Check sheet for the modelled part. Datum: model origin and axes. Units: mm. Face numbers are marked on the shaded views. A direction names the side the tool comes from. Give positions to 0.01 mm unless a question says otherwise; leave off trailing zeros. Order: outer loops, then holes, each group sorted by start corner. A loop starts at its lowest first (then second) coordinate and runs counter-clockwise, first axis right, second up.
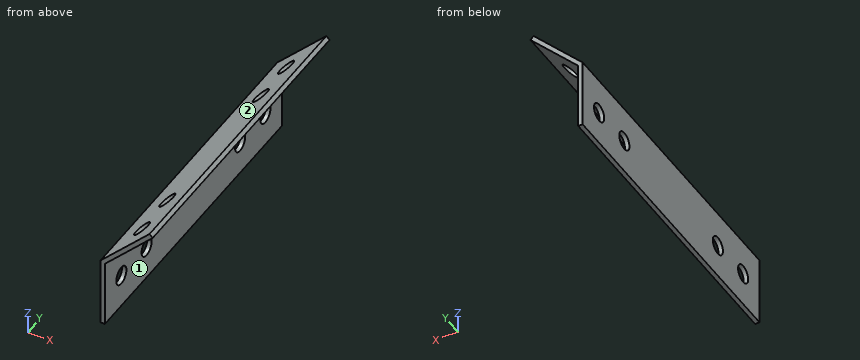
from build123d import *

# Parameters (mm, degrees)
EXTRUSION1_DEPTH = 70
EXTRUSION2_REACH = 3
ESQUISSE2_R      = 2
EXTRUSION3_REACH = 10.707
ESQUISSE3_R      = 2


with BuildPart() as part:
    # Esquisse1 → Extrusion1 (new body)
    with BuildSketch(Plane(origin=(0, 0, 0), x_dir=(1, 0, 0), z_dir=(0, 1, 0))):
        Polygon((0, 0), (0, 15.414213562), (1, 15.414213562), (1, 0.414213562), (11.606601718, -10.192388155), (10.899494937, -10.899494937), align=None)
    extrude(amount=EXTRUSION1_DEPTH)

    # Esquisse2 → Extrusion2 (cut, up to next)
    with BuildSketch(Plane(origin=(1, 0, 0), x_dir=(0, 0, -1), z_dir=(1, 0, 0)), mode=Mode.PRIVATE) as extrusion2_sk1:
        with Locations((7.914213562, 16.5)):
            Circle(ESQUISSE2_R)
    extrusion2_tool1 = extrude(extrusion2_sk1.sketch, amount=-EXTRUSION2_REACH, mode=Mode.PRIVATE) & part.part
    add(extrusion2_tool1.solids().sort_by_distance((1, 16.5, -7.914214))[0], mode=Mode.SUBTRACT)
    # Esquisse2 → Extrusion2 (cut, up to next)
    with BuildSketch(Plane(origin=(1, 0, 0), x_dir=(0, 0, -1), z_dir=(1, 0, 0)), mode=Mode.PRIVATE) as extrusion2_sk2:
        with Locations((7.914213562, 6.5)):
            Circle(ESQUISSE2_R)
    extrusion2_tool2 = extrude(extrusion2_sk2.sketch, amount=-EXTRUSION2_REACH, mode=Mode.PRIVATE) & part.part
    add(extrusion2_tool2.solids().sort_by_distance((1, 6.5, -7.914214))[0], mode=Mode.SUBTRACT)
    # Esquisse2 → Extrusion2 (cut, up to next)
    with BuildSketch(Plane(origin=(1, 0, 0), x_dir=(0, 0, -1), z_dir=(1, 0, 0)), mode=Mode.PRIVATE) as extrusion2_sk3:
        with Locations((7.914213562, 53.5)):
            Circle(ESQUISSE2_R)
    extrusion2_tool3 = extrude(extrusion2_sk3.sketch, amount=-EXTRUSION2_REACH, mode=Mode.PRIVATE) & part.part
    add(extrusion2_tool3.solids().sort_by_distance((1, 53.5, -7.914214))[0], mode=Mode.SUBTRACT)
    # Esquisse2 → Extrusion2 (cut, up to next)
    with BuildSketch(Plane(origin=(1, 0, 0), x_dir=(0, 0, -1), z_dir=(1, 0, 0)), mode=Mode.PRIVATE) as extrusion2_sk4:
        with Locations((7.914213562, 63.5)):
            Circle(ESQUISSE2_R)
    extrusion2_tool4 = extrude(extrusion2_sk4.sketch, amount=-EXTRUSION2_REACH, mode=Mode.PRIVATE) & part.part
    add(extrusion2_tool4.solids().sort_by_distance((1, 63.5, -7.914214))[0], mode=Mode.SUBTRACT)

    # Esquisse3 → Extrusion3 (cut, up to next)
    with BuildSketch(Plane(origin=(0.707106781, 0, -0.707106781), x_dir=(-0.707106781, 0, -0.707106781), z_dir=(0.707106781, 0, -0.707106781)), mode=Mode.PRIVATE) as extrusion3_sk1:
        with Locations((-7.914213562, 53.5)):
            Circle(ESQUISSE3_R)
    extrusion3_tool1 = extrude(extrusion3_sk1.sketch, amount=-EXTRUSION3_REACH, mode=Mode.PRIVATE) & part.part
    add(extrusion3_tool1.solids().sort_by_distance((6.303301, 53.5, 4.889087))[0], mode=Mode.SUBTRACT)
    # Esquisse3 → Extrusion3 (cut, up to next)
    with BuildSketch(Plane(origin=(0.707106781, 0, -0.707106781), x_dir=(-0.707106781, 0, -0.707106781), z_dir=(0.707106781, 0, -0.707106781)), mode=Mode.PRIVATE) as extrusion3_sk2:
        with Locations((-7.914213562, 63.5)):
            Circle(ESQUISSE3_R)
    extrusion3_tool2 = extrude(extrusion3_sk2.sketch, amount=-EXTRUSION3_REACH, mode=Mode.PRIVATE) & part.part
    add(extrusion3_tool2.solids().sort_by_distance((6.303301, 63.5, 4.889087))[0], mode=Mode.SUBTRACT)
    # Esquisse3 → Extrusion3 (cut, up to next)
    with BuildSketch(Plane(origin=(0.707106781, 0, -0.707106781), x_dir=(-0.707106781, 0, -0.707106781), z_dir=(0.707106781, 0, -0.707106781)), mode=Mode.PRIVATE) as extrusion3_sk3:
        with Locations((-7.914213562, 6.5)):
            Circle(ESQUISSE3_R)
    extrusion3_tool3 = extrude(extrusion3_sk3.sketch, amount=-EXTRUSION3_REACH, mode=Mode.PRIVATE) & part.part
    add(extrusion3_tool3.solids().sort_by_distance((6.303301, 6.5, 4.889087))[0], mode=Mode.SUBTRACT)
    # Esquisse3 → Extrusion3 (cut, up to next)
    with BuildSketch(Plane(origin=(0.707106781, 0, -0.707106781), x_dir=(-0.707106781, 0, -0.707106781), z_dir=(0.707106781, 0, -0.707106781)), mode=Mode.PRIVATE) as extrusion3_sk4:
        with Locations((-7.914213562, 16.5)):
            Circle(ESQUISSE3_R)
    extrusion3_tool4 = extrude(extrusion3_sk4.sketch, amount=-EXTRUSION3_REACH, mode=Mode.PRIVATE) & part.part
    add(extrusion3_tool4.solids().sort_by_distance((6.303301, 16.5, 4.889087))[0], mode=Mode.SUBTRACT)


solid = part.part
1) Section check B-B, the plane z = -12. Record the cut outline in (x, y).
Recorded:
outline: (0, 0) - (1, 0) - (1, 70) - (0, 70) - close
2) Material ranges on L1, parallel to X at y = 12, z = -12; L2, parallel to Z at x = 1.5, y = 20.5; L3, parallel to Z at x = 2, y = 14.5, recorded low to high.
Recorded:
L1: x = 0 to 1
L2: z = 0.09 to 1.5
L3: z = 0.59 to 2
3) Section check D-D, the plane y = 44.5. Record the cut outline in (x, z), then the cut area to 3 significant figures.
Recorded:
outline: (0, -15.41) - (1, -15.41) - (1, -0.41) - (11.61, 10.19) - (10.9, 10.9) - (0, 0) - close
area: 30.4 mm2
4) Section check C-C, the plane x = 5.75. State how many separate pieces and enclosed holes the cut face has, then the cut area to 3 significant figures.
Recorded:
separate pieces: 5
enclosed holes: 0
area: 76.8 mm2
5) Section check A-A, the plane y = 6.5. Record the cut outline in (x, z), then the cut area to 3 significant figures.
Recorded:
outline: (0, -15.41) - (1, -15.41) - (1, -9.91) - (0, -9.91) - close; (0, -5.91) - (1, -5.91) - (1, -0.41) - (4.89, 3.47) - (4.18, 4.18) - (0, 0) - close; (7.01, 7.01) - (7.72, 6.3) - (11.61, 10.19) - (10.9, 10.9) - close
area: 22.4 mm2
6) Set-up check for the marked faces 1 and 2: record each of +Z, -Z, +X, -X, +Y, -Y from which the full face is reachable in a straight line by a thin tool's end or side.
Recorded:
face 1: -Z, +X, +Y, -Y
face 2: +Z, -X, +Y, -Y
7) Depth check by flat-ended pin: pin 1 Ø4 at (y, z) = (24.5, -3) entering from -X; pin 2 Ø6 at (x, y) = (4, 51) entering from +Z; pin 3 Ø3 at (y, z) = (25.5, 4) entering from +X; pin 4 Ø6.5 at (y, z) = (63.5, -7.91) entering from +X. Enter the tip coordinate at first touch or a pass-through.
Recorded:
pin 1: stops at x = 0
pin 2: stops at z = 7
pin 3: stops at x = 6.91
pin 4: stops at x = 1
